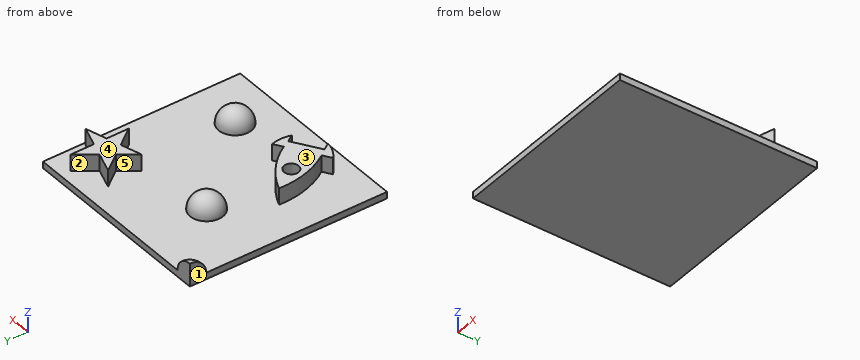
from build123d import *

# Parameters (mm, degrees)
F0_W     = 152.4
F0_H     = 152.4
F2_DEPTH = 5.08
F5_ANGLE = 90
F6_ANGLE = 180
F7_ANGLE = 180
F4_R     = 5.6279425354
F8_DEPTH = 12.7


with BuildPart() as f2:
    # F0 (on Top) → F2 (new body)
    with BuildSketch(Plane.XY):
        Rectangle(F0_W, F0_H)
    extrude(amount=F2_DEPTH)

    # F4 (on face) → F5 (revolve)
    with BuildSketch(Plane.XY.offset(5.08)):
        with BuildLine():
            Line((-76.2, 76.2), (-76.2, 63.5))
            ThreePointArc((-76.2, 63.5), (-67.2197438789, 67.2197438789), (-63.5, 76.2))
            Line((-63.5, 76.2), (-76.2, 76.2))
        make_face()
    revolve(axis=Axis((-76.2, 0, 5.08), (0, -1, 0)), revolution_arc=F5_ANGLE)

    # F4 (on face) → F6 (revolve)
    with BuildSketch(Plane.XY.offset(5.08)):
        with BuildLine():
            Line((24.2210256122, -43.0185761551), (49.6210256122, -43.0185761551))
            ThreePointArc((49.6210256122, -43.0185761551), (36.9210256122, -30.3185761551), (24.2210256122, -43.0185761551))
        make_face()
    revolve(axis=Axis((36.9210256122, -43.0185761551, 5.08), (1, 0, 0)), revolution_arc=F6_ANGLE)

    # F4 (on face) → F7 (revolve)
    with BuildSketch(Plane.XY.offset(5.08)):
        with BuildLine():
            ThreePointArc((-10.9549105823, 24.090602994), (-23.6549105823, 36.790602994), (-36.3549105823, 24.090602994))
            Line((-36.3549105823, 24.090602994), (-10.9549105823, 24.090602994))
        make_face()
    revolve(axis=Axis((-23.6549105823, 24.090602994, 5.08), (1, 0, 0)), revolution_arc=F7_ANGLE)

    # F4 (on face) → F8 (join)
    with BuildSketch(Plane.XY.offset(5.08)):
        Polygon((47.570896451, 53.8189061847), (31.3873370203, 59.2746157033), (41.5168850169, 45.6796259761), (31.9747962058, 32.8508205712), (47.7112500038, 37.36609329), (58.2554601133, 23.2145804912), (58.2554601133, 40.3915515578), (74.0002126055, 44.9092054273), (58.2554601133, 50.2169868464), (58.2554601133, 68.1837052107), align=None)
        with BuildLine():
            ThreePointArc((-35.3100343123, -56.0667765948), (-33.4447317203, -58.6502472307), (-31.4584446243, -61.1419008701))
            Line((-31.4584446243, -61.1419008701), (-11.2081296183, -48.2286563014))
            ThreePointArc((-11.2081296183, -48.2286563014), (-12.6293719871, -45.3766842792), (-14.1848974706, -42.5956746142))
            ThreePointArc((-14.1848974706, -42.5956746142), (-28.2369814707, -25.8469443278), (-46.9412207919, -14.5273832774))
            ThreePointArc((-46.9412207919, -14.5273832774), (-44.5680834417, -36.2609805423), (-35.3100343123, -56.0667765948))
        make_face()
        with Locations((-35.3753649504, -32.6647478149)):
            Circle(F4_R, mode=Mode.SUBTRACT)
        with BuildLine():
            ThreePointArc((-14.1848974706, -42.5956746142), (-12.6293719871, -45.3766842792), (-11.2081296183, -48.2286563014))
            Line((-11.2081296183, -48.2286563014), (-7.7939508483, -53.5827092826))
            ThreePointArc((-7.7939508483, -53.5827092826), (-6.5000191862, -46.0352288655), (-7.7248563313, -38.4762280214))
            Line((-7.7248563313, -38.4762280214), (-14.1848974706, -42.5956746142))
        make_face()
        with BuildLine():
            Line((-28.0442658543, -66.4959538513), (-31.4584446243, -61.1419008701))
            ThreePointArc((-31.4584446243, -61.1419008701), (-33.4447317203, -58.6502472307), (-35.3100343123, -56.0667765948))
            Line((-35.3100343123, -56.0667765948), (-41.7700754515, -60.1862231876))
            ThreePointArc((-41.7700754515, -60.1862231876), (-35.4331949634, -64.4853702509), (-28.0442658543, -66.4959538513))
        make_face()
    extrude(amount=F8_DEPTH)


solid = f2.part
Geometry check sheet. Reference: the model listing, model coordinates, mm. Face numbers are marked on the shaded views. A direction names the side the tool comes from. Round coordinates to 2 decimals unless told otherwise and drop trailing zeros. Order: outer loops, then holes, each group sorted by start corner. A loop starts at its lowest first (then second) coordinate and runs counter-clockwise, first axis right, second up. Notation, with made-up numbers: M -24,18.5 L -12,18.5 A11 cw -12,25.5 Z; hole C 52.25,1 d1. An arc over 180 degrees is marked long. Answer in a Markdown table with one row per item.
(1) Sectioned sample at A-A, the plane z = 15. Record the cut outline in (x, y).
Responses:
| item | result |
|---|---|
| outline | M -76.2,68.27 A7.93 ccw -68.27,76.2 L -76.2,76.2 Z; M -46.94,-14.53 A66.85 ccw -35.31,-56.07 L -41.77,-60.19 A23.28 ccw -28.04,-66.5 L -31.46,-61.14 L -11.21,-48.23 L -7.79,-53.58 A23.28 ccw -7.72,-38.48 L -14.18,-42.6 A66.85 ccw Z; C -23.65,24.09 d15.86; C 36.92,-43.02 d15.86; M 31.39,59.27 L 41.52,45.68 L 31.97,32.85 L 47.71,37.37 L 58.26,23.21 L 58.26,40.39 L 74,44.91 L 58.26,50.22 L 58.26,68.18 L 47.57,53.82 Z; hole C -35.38,-32.66 d11.26 |
(2) Sectioned sample at C-C, the plane x = -65.5. Record the cut outline in (y, z), and give its area (3 significant figures).
Responses:
| item | result |
|---|---|
| outline | M -76.2,0 L 76.2,0 L 76.2,11.92 A6.84 ccw 69.36,5.08 L -76.2,5.08 Z |
| area | 811 mm² |
(3) Draft check along X on the marked faces 1, 2 and 3. Enter one of: released by +X, released by -X, zero draft, split by the parting line, or undercut.
Responses:
| item | result |
|---|---|
| face 1 | released by -X |
| face 2 | undercut |
| face 3 | zero draft |
(4) Scan lines: probe 1 along Y at (x, z) = (-40, 16.75); probe 2 along Y at (x, z) = (33, 8); probe 3 along Z at (x, y) = (-57, 2). Record each from-to range of solid material in increasing order. Write a range as from..to.
Responses:
| item | result |
|---|---|
| probe 1 | y = -61.71..-59.06, -48.11..-35.87, -29.46..-17.77 |
| probe 2 | y = -54.74..-31.3, 33.14..34.23, 57.11..58.73 |
| probe 3 | z = 0..5.08 |
(5) Sectioned sample at B-B, the plane y = -64. Record the cut outline in (x, z), and give its area (3 significant figures).
Responses:
| item | result |
|---|---|
| outline | M -76.2,0 L 76.2,0 L 76.2,5.08 L -29.64,5.08 L -29.64,17.78 L -36.43,17.78 L -36.43,5.08 L -76.2,5.08 Z |
| area | 860 mm² |
(6) Go/stop test with flat-tipped pins: P1, Ø2, axis at x = 56, z = 11.5, coming from the +Y side; P2, Ø3.5, axis at x = -38, y = -35, coming from the +Z side; P3, Ø1.5, axis at x = 59.5, z = 13.5, coming from the -Y side. Record where each tip stops, or that it passes through.
Responses:
| item | result |
|---|---|
| P1 | stops at y = 66.5 |
| P2 | stops at z = 5.08 |
| P3 | stops at y = 40.53 |
(7) Tool access check on the marked faces 4 and 5. Record the directions out of +Z, -Z, +X, -X, +Y, -Y that give a thin tool (end or side, any length) a straight path to the whole face; none if there is none.
Responses:
| item | result |
|---|---|
| face 4 | +Z, +X, -X, +Y, -Y |
| face 5 | +Z |
(8) Sectioned sample at D-D, the plane x = 34.5. Record the cut outline in (y, z).
Responses:
| item | result |
|---|---|
| outline | M -76.2,0 L 76.2,0 L 76.2,5.08 L 58.23,5.08 L 58.23,17.78 L 55.1,17.78 L 55.1,5.08 L 36.25,5.08 L 36.25,17.78 L 33.58,17.78 L 33.58,5.08 L -30.55,5.08 A12.47 ccw -55.49,5.08 L -76.2,5.08 Z |
